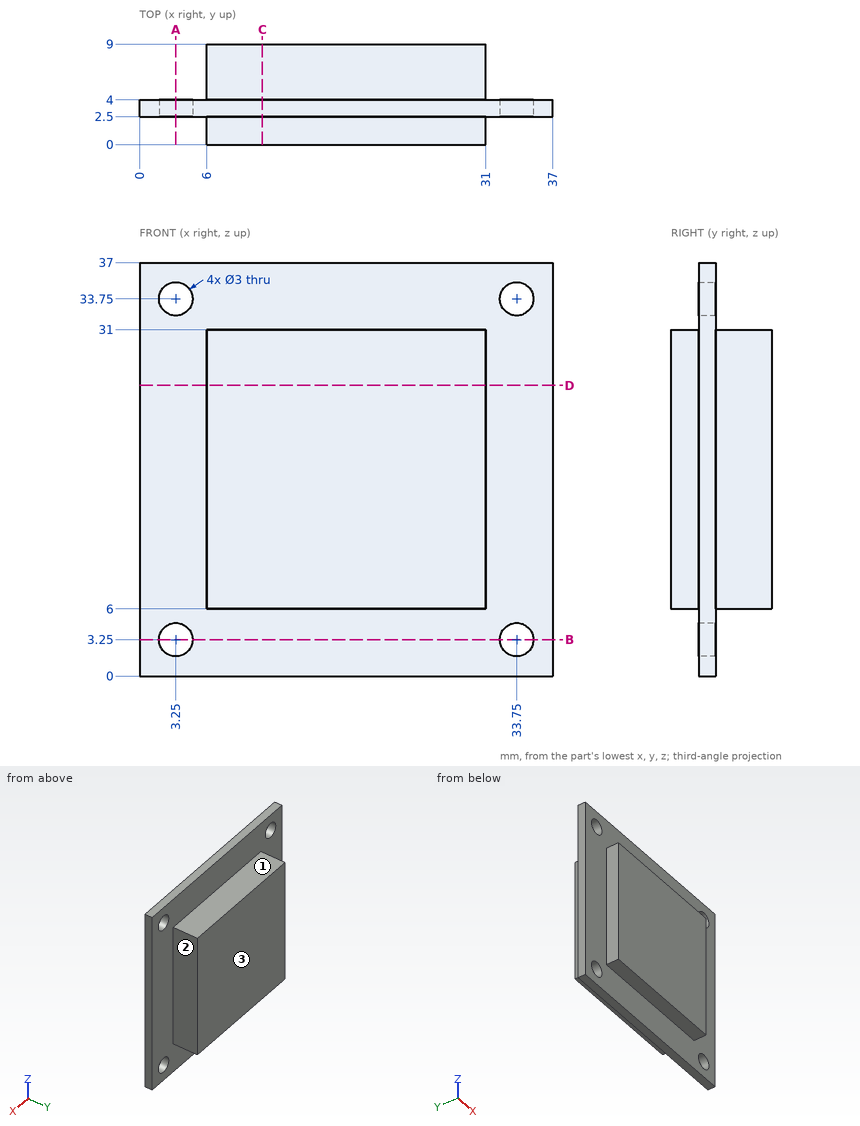
Input: dimensioned drawing with shaded views. Units: mm. Origin: part minimum x, y, z. A direction names the side the tool comes from. Give positions to 0.01 mm unless a question says otherwise; leave off trailing zeros. Order: outer loops, then holes, each group sorted by start corner. A loop starts at its lowest first (then second) coordinate and runs counter-clockwise, first axis right, second up. Notation, with made-up numbers: (-4, 53) -> (48, 53) arc R17 cw to (48, 85) -> close; hole circle Ø2 at (-38.75, -14). An arc over 180 degrees is marked (long way). Use a Markdown table: item, result.
1) Contact query for flat-ended pins moving along their axis: P1, Ø4, axis at y = 1, z = 28.5, coming from the -X side; P2, Ø0.8, axis at x = 23, y = 2, coming from the +Z side; P3, Ø4, axis at x = 3.25, z = 33.75, coming from the -Y side; P4, Ø2, axis at x = 24.5, y = 0.5, coming from the -Z side. Output: stop coordinate, or through.
Answer list:
| item | result |
|---|---|
| P1 | x = 0 |
| P2 | z = 31 |
| P3 | y = 2.5 |
| P4 | z = 6 |
2) Section query B-B, the plane z = 3.25. Return the cut outline in (x, y), then the cut area to 3 significant figures.
Answer list:
| item | result |
|---|---|
| outline | (0, 2.5) -> (1.75, 2.5) -> (1.75, 4) -> (0, 4) -> close; (4.75, 2.5) -> (32.25, 2.5) -> (32.25, 4) -> (4.75, 4) -> close; (35.25, 2.5) -> (37, 2.5) -> (37, 4) -> (35.25, 4) -> close |
| area | 46.5 mm² |
3) Section query D-D, the plane z = 26. Return the cut outline in (x, y), then the cut area to 3 significant figures.
Answer list:
| item | result |
|---|---|
| outline | (0, 2.5) -> (6, 2.5) -> (6, 0) -> (31, 0) -> (31, 2.5) -> (37, 2.5) -> (37, 4) -> (31, 4) -> (31, 9) -> (6, 9) -> (6, 4) -> (0, 4) -> close |
| area | 243 mm² |
4) Reachability of the marked faces 1, 2 and 3 from +Z, -Z, +X, -X, +Y, -Y: full face, straight path, thin tool, end or side. Return the list, or none.
Answer list:
| item | result |
|---|---|
| face 1 | +Z, +X, -X, +Y |
| face 2 | +Z, -Z, +X, +Y |
| face 3 | +Z, -Z, +X, -X, +Y |
5) Section query A-A, the plane x = 3.25. Return the cut outline in (y, z), then the cut area to 3 significant figures.
Answer list:
| item | result |
|---|---|
| outline | (2.5, 0) -> (4, 0) -> (4, 1.75) -> (2.5, 1.75) -> close; (2.5, 4.75) -> (4, 4.75) -> (4, 32.25) -> (2.5, 32.25) -> close; (2.5, 35.25) -> (4, 35.25) -> (4, 37) -> (2.5, 37) -> close |
| area | 46.5 mm² |
6) Ray query, line 1 along X through (y, z) = (3.6, 3.25); line 2 along Z through (x, y) = (20, 5); line 3 along Y through (x, z) = (35.5, 5). Return the intervals inside material, ascending. Write a range as [from, to].
Answer list:
| item | result |
|---|---|
| line 1 | [0, 1.75], [4.75, 32.25], [35.25, 37] |
| line 2 | [6, 31] |
| line 3 | [2.5, 4] |
7) Section query C-C, the plane x = 11. Return the cut outline in (y, z), then the cut area to 3 significant figures.
Answer list:
| item | result |
|---|---|
| outline | (0, 6) -> (2.5, 6) -> (2.5, 0) -> (4, 0) -> (4, 6) -> (9, 6) -> (9, 31) -> (4, 31) -> (4, 37) -> (2.5, 37) -> (2.5, 31) -> (0, 31) -> close |
| area | 243 mm² |
